Here's how the part is built. I have some questions about the finished solid (model axes, mm). A direction names the side the tool comes from. Give positions to 0.01 mm unless a question says otherwise; leave off trailing zeros. Loops run counter-clockwise (first coordinate to the right, second up) from the corner with the lowest first, then second, coordinate; pieces in that order, holes last.
Q1. If we section it at A-A (y = 0): Please give me the cut outline in (x, z) (3 decimals).
Q2. If we section it at B-B (x = 19): Please give me the cut outline in (y, z) (3 decimals), plus the area to 3 significant figures.
Q3. If we section it at C-C (z = 9): Please give me the cut outline in (x, y) (3 decimals), plus the area to 3 significant figures.
Q4. If we section it at D-D (z = 35): Please give me the cut outline in (x, y) (3 decimals).
Q5. We'd pull the mould along Z, two halves only. Please class faces 3 (the face through (63, -1, 0)), 4 (the face through (14.55, 9.516, 38.519)), 5 (the face through (0, -1, 26)): +Z half, -Z half, draft (parallel to the pull), parting line (faces both ways), or undercut.
Q6. Will these pins go through, and if not, where does the flat tip stop? P1, Ø25, axis at x = 38.1, y = 0, coming from the +Z side; P2, Ø2, axis at x = 98, y = 20.5, coming from the +Z side; P3, Ø12, axis at y = 16, z = 39.5, coming from the +X side.
Q7. For faces 1 (the face through (102, -1, 25.4)), 2 (the face through (48, 38.1, 20)), which set-ups out of +Z, -Z, +X, -X, +Y, -Y let a thin tool reach every point of the face, with its end or its side?
Q8. I need wall thicknesses on line 1 (Y direction, x = 67, z = 38.1) (3 decimals); line 2 (Z direction, x = 49, y = 0) (3 decimals); line 3 (Z direction, x = 120, y = -8). Which ranges of each line are inside material? Lowest first, please.
from build123d import *

# Parameters (mm, degrees)
F1_DEPTH = 38.1
F3_D     = 19.05
F5_D     = 19.05


with BuildPart() as f1:
    # F0 (on Front) → F1 (new body, symmetric)
    with BuildSketch(Plane.XZ):
        Polygon((0, 50.8), (0, 0), (127, 0), (127, 25.4), (76.2, 25.4), (76.2, 50.8), align=None)
    extrude(amount=F1_DEPTH, both=True)

    # F3 (through all)
    with Locations(Plane.XY.offset(50.8)):
        with Locations((38.1, 0)):
            Hole(F3_D / 2)

    # F5 (through all)
    with Locations(Plane.YZ.offset(76.2)):
        with Locations((0, 38.1)):
            Hole(F5_D / 2)


solid = f1.part
Check sheet entries:
1. outline: (0, 0) - (28.575, 0) - (28.575, 28.575) - (0, 28.575) - close; (0, 47.625) - (28.575, 47.625) - (28.575, 50.8) - (0, 50.8) - close; (47.625, 0) - (127, 0) - (127, 25.4) - (76.2, 25.4) - (76.2, 28.575) - (47.625, 28.575) - close; (47.625, 47.625) - (76.2, 47.625) - (76.2, 50.8) - (47.625, 50.8) - close
2. outline: (-38.1, 0) - (38.1, 0) - (38.1, 50.8) - (-38.1, 50.8) - close; hole circle Ø19.05 at (0, 38.1)
2. area: 3,590 mm2
3. outline: (0, -38.1) - (127, -38.1) - (127, 38.1) - (0, 38.1) - close; hole circle Ø19.05 at (38.1, 0)
3. area: 9,390 mm2
4. outline: (0, -38.1) - (76.2, -38.1) - (76.2, -9.006) - (41.2, -9.006) arc R9.525 cw to (35, -9.006) - (0, -9.006) - close; (0, 9.006) - (35, 9.006) arc R9.525 cw to (41.2, 9.006) - (76.2, 9.006) - (76.2, 38.1) - (0, 38.1) - close
5. face 3: -Z half
5. face 4: undercut
5. face 5: draft
6. P1: stops at z = 50.8
6. P2: stops at z = 25.4
6. P3: stops at x = 76.2
7. face 1: +Z, +X, +Y, -Y
7. face 2: +Z, -Z, +X, -X, +Y
8. line 1: y = -38.1 to -9.525, 9.525 to 38.1
8. line 2: z = 0 to 28.575, 47.625 to 50.8
8. line 3: z = 0 to 25.4
